Geometry check sheet. Reference: drawing and pictorial views, mm from the part's lowest x, y, z. A direction names the side the tool comes from. Round coordinates to 2 decimals unless told otherwise and drop trailing zeros. Loops run counter-clockwise (first coordinate to the right, second up) from the corner with the lowest first, then second, coordinate; pieces in that order, holes last. Notation, with made-up numbers: (-35.75, -11) - (-4.75, -11) arc R29 ccw to (-4.75, 18) - close; hole circle Ø10 at (52, 1.25). An arc over 180 degrees is marked (long way). Answer as CSV lines item,"result". Start each with the question number.
1) Access from +Z, -Z, +X, -X, +Y, -Y to the whole of each face (thin tool, end or side, straight path). Record for the marked faces 1 and 2.
2) Cross-section at C-C on x = 4.5. Record the boundary of the cut face in (y, z) (1 decimal).
3) Cross-section at A-A on y = 24. Record the boundary of the cut face in (x, z) (1 decimal).
4) Thickness scan on line 1 along Y through (x, z) = (25.5, 1.45); line 2 along Y through (x, z) = (31, 0.45) (1 decimal). Record the ranges inside material, lowest first.
5) Draft check along X on the marked faces 3 and 4. Enter one of: released by +X, released by -X, zero draft, split by the parting line, or undercut.
6) Depth check by flat-ended pin: P1, Ø6, axis at x = 11, y = 22, coming from the +Z side; P2, Ø1, axis at x = 26, z = 0.5, coming from the -Y side. Enter the tip coordinate at first touch or a pass-through.
7) Cross-section at D-D on z = 2.4. Record the boundary of the cut face in (x, y).
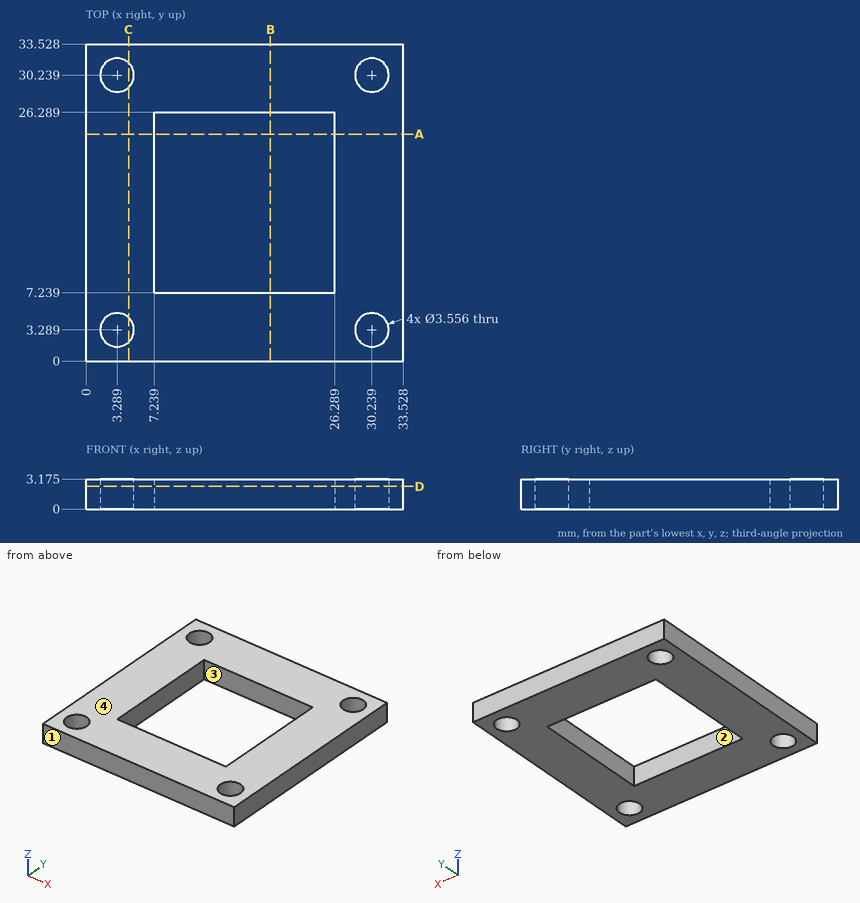
Answer block:
1,face 1,"+Z, -Z, +X, -X, -Y"
1,face 2,"+Z, -Z"
2,outline,"(0, 0) - (2, 0) - (2, 3.2) - (0, 3.2) - close; (4.6, 0) - (28.9, 0) - (28.9, 3.2) - (4.6, 3.2) - close; (31.5, 0) - (33.5, 0) - (33.5, 3.2) - (31.5, 3.2) - close"
3,outline,"(0, 0) - (7.2, 0) - (7.2, 3.2) - (0, 3.2) - close; (26.3, 0) - (33.5, 0) - (33.5, 3.2) - (26.3, 3.2) - close"
4,line 1,"y = 0 to 7.24, 26.29 to 33.53"
4,line 2,"y = 0 to 1.7, 4.9 to 28.6, 31.8 to 33.5"
5,face 3,"undercut"
5,face 4,"zero draft"
6,P1,"passes through"
6,P2,"stops at y = 0"
7,outline,"(0, 0) - (33.53, 0) - (33.53, 33.53) - (0, 33.53) - close; hole circle Ø3.56 at (3.29, 3.29); hole circle Ø3.56 at (3.29, 30.24); hole (7.24, 7.24) - (26.29, 7.24) - (26.29, 26.29) - (7.24, 26.29) - close; hole circle Ø3.56 at (30.24, 3.29); hole circle Ø3.56 at (30.24, 30.24)"
